Part model, mm, in its own coordinate system. Face numbers are marked on the shaded views. Give positions to 0.01 mm unless a question says otherwise; leave off trailing zeros. Order: outer loops, then holes, each group sorted by start corner. A loop starts at its lowest first (then second) coordinate and runs counter-clockwise, first axis right, second up. Notation, with made-up numbers: (-18, 5.25) - (11, 5.25) arc R5 cw to (11, 13.25) - close; hole circle Ø7 at (24.5, 1.25). An arc over 180 degrees is marked (long way). One line per item, written item: value.
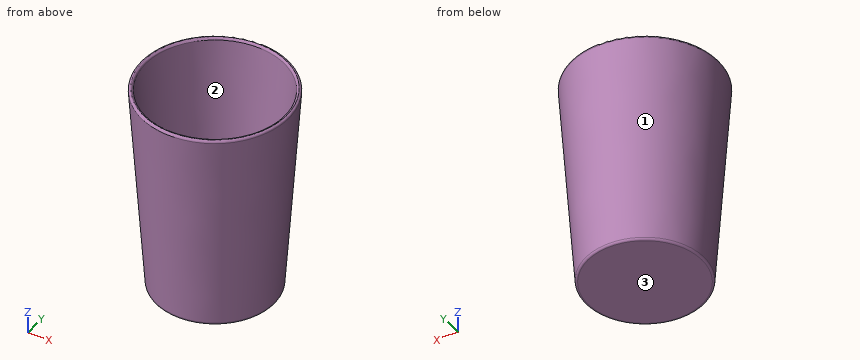
```python
from build123d import *

# Parameters (mm, degrees)
F2_R = 0.99999


# Not quite as in the source:
# - a fillet or chamfer is up to 0.001 mm smaller than in the source, because OpenCascade refuses the exact size


with BuildPart() as f1:
    # F0 (on Front) → F1 (revolve)
    with BuildSketch(Plane.XZ):
        Polygon((-31.9951162038, 79.5454481112), (-34, 79.5454481112), (-27.2870260534, -16.4545518888), (0, -16.4545518888), (0, -14.4545518888), (-25.4219958811, -14.4545518888), align=None)
    revolve(axis=Axis((0, 0, -15.4545518888), (0, 0, 1)))

    # F2 (radius 1 in the source; OpenCascade refuses exactly that, so slightly less here)
    f2_edges = [f1.edges().sort_by_distance(p)[0] for p in [
        (27.287026, 0, -16.454552),
        (34, 0, 79.545448),
        (31.995116, 0, 79.545448),
    ]]
    fillet(f2_edges, radius=F2_R)


solid = f1.part
```
1) Drill centre lines: line 1 along Y through (x, z) = (-21.5, -2.5); line 2 along X through (y, z) = (0, 56); line 3 along Z through (x, y) = (20.5, 2.5). Where is each one in solid material? Low to high. Write a range as from..to.
Outcome:
line 1: y = -18.34..-15.07, 15.07..18.34
line 2: x = -32.35..-30.35, 30.35..32.35
line 3: z = -16.45..-14.45
2) Pin check, flat tips, straight feed: pin 1 (8 mm diameter, centred on x = 9, z = 37.5, fed in from +Y); pin 2 (1.5 mm diameter, centred on x = -19, z = 43.5, fed in from -Y); pin 3 (1.5 mm diameter, centred on y = 9.5, z = 8, fed in from +X). Stop position of each tip, or through.
Outcome:
pin 1: stops at y = 30.71
pin 2: stops at y = -25.65
pin 3: stops at x = 27.65
3) Cut at D-D, the plane z = 21. Give the cut face in (x, y).
Outcome:
outline: circle Ø59.81 at (0, 0); hole circle Ø55.8 at (0, 0)
4) Mould opens along Y. For the marked faces 1, 2 and 3 say: released by +Y, released by -Y, zero draft, split by the parting line, or undercut.
Outcome:
face 1: split by the parting line
face 2: undercut
face 3: zero draft
5) Cut at C-C, the plane z = 73. Give the cut face in (x, y).
Outcome:
outline: circle Ø67.08 at (0, 0); hole circle Ø63.07 at (0, 0)
